The model under review builds one solid part; all positions refer to its coordinate system, in mm. Give positions to 0.01 mm unless a question says otherwise; leave off trailing zeros. Loops run counter-clockwise (first coordinate to the right, second up) from the corner with the lowest first, then second, coordinate; pieces in that order, holes last. Notation, with made-up numbers: M 35.25,56.5 L 53.25,56.5 A27 cw 53.25,84.5 Z; hole C -15.5,-20 d10. An arc over 180 degrees is marked long. Return JSON: item names as keys, results as strings.
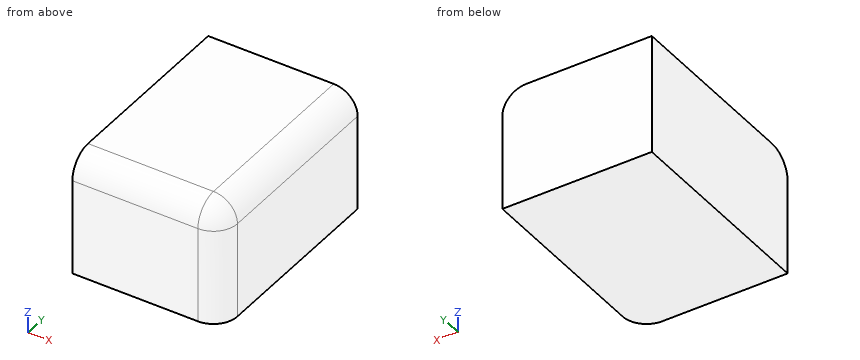
```python
from build123d import *

# Parameters (mm, degrees)
F0_W        = 31.75
F0_H        = 25.4
F1_DEPTH    = 44.196
F2_R        = 5.08
F3_T1_DEPTH = 33.02
F3_S5_W     = 5.08
F3_S5_H     = 5.08
F3_T6_DEPTH = 5.08


# Not quite as in the source:
# - a fillet or chamfer that OpenCascade refuses, or shapes differently, is made with other operations: its cross-section is extruded or revolved along the edge and cut away or added


with BuildPart() as f1:
    # F0 (on Front) → F1 (new body)
    with BuildSketch(Plane.XZ):
        with Locations((3.175, 0)):
            Rectangle(F0_W, F0_H)
    extrude(amount=F1_DEPTH)

    # F2
    f2_edges = [f1.edges().sort_by_distance(p)[0] for p in [
        (3.175, -44.196, 12.7),
        (19.05, -22.098, 12.7),
    ]]
    fillet(f2_edges, radius=F2_R)

    # F3: fillet of radius 5.08 on 1 edges, made by hand

    # F3_s2 → F3_t1 (cut)
    with BuildSketch(Plane.XY.offset(-25.4)):
        with BuildLine():
            ThreePointArc((13.97, -44.196), (17.5621024484, -42.7081024484), (19.05, -39.116))
            Line((19.05, -39.116), (19.05, -44.196))
            Line((19.05, -44.196), (13.97, -44.196))
        make_face()
    extrude(amount=F3_T1_DEPTH, mode=Mode.SUBTRACT)


with BuildPart() as f3_tool4:
    # F3_s5 → F3_t6 (new body)
    with BuildSketch(Plane.XZ.offset(39.116)):
        with Locations((16.51, 10.16)):
            Rectangle(F3_S5_W, F3_S5_H)
    extrude(amount=F3_T6_DEPTH)

    # F3_s7 → F3_t8 (revolve, cut)
    with BuildSketch(Plane(origin=(13.97, -39.116, 7.62), x_dir=(-0.7071067812, 0, -0.7071067812), z_dir=(-0.7071067812, 0, 0.7071067812))):
        with BuildLine():
            ThreePointArc((0, -5.08), (5.08, 0), (0, 5.08))
            Line((0, 5.08), (0, -5.08))
        make_face()
    revolve(axis=Axis((13.97, -39.116, 7.62), (0, -1, 0)), mode=Mode.SUBTRACT)


with BuildPart() as f1_1:
    add(f1.part)

    # F3_t3: cut F3_tool4
    add(f3_tool4.part, mode=Mode.SUBTRACT)


solid = f1_1.part
```
1) Wall thickness on L1, parallel to Z at x = 14.5, y = -40.5; L2, parallel to Y at x = -6, z = 8; L3, parallel to Y at x = -4.5, z = 9: over which ranges is each line inside the solid? List them lowest first. Write a range as from..to.
From the geometry:
{"L1": "-12.7..12.48", "L2": "-44.18..0", "L3": "-44..0"}
2) Consider section A-A on z = 10. Write out the cut boundary in (x, y).
From the geometry:
{"outline": "M -12.7,-43.6 L 13.97,-43.6 A4.49 ccw 18.46,-39.12 L 18.46,0 L -12.7,0 Z"}
3) Insertion check: pin 1 (1.5 mm diameter, centred on x = 15, z = 6.5, fed in from +Y). The pin has a flat end and moves straight along its axis. Give the tip position at first contact, or say it passes through.
From the geometry:
{"pin 1": "y = 0"}
